from build123d import *

# Parameters (mm, degrees)
SKETCH1_W           = 110
SKETCH1_H           = 30
BOSS_EXTRUDE1_DEPTH = 6
SKETCH2_R           = 2
CUT_EXTRUDE1_DEPTH  = 10


with BuildPart() as part:
    # Sketch1 → Boss-Extrude1 (new body)
    with BuildSketch(Plane(origin=(0, 0, 0), x_dir=(1, 0, 0), z_dir=(0, 1, 0))):
        with Locations((-47.510460251, 50.167364017)):
            Rectangle(SKETCH1_W, SKETCH1_H)
    extrude(amount=BOSS_EXTRUDE1_DEPTH)

    # Sketch2 → Cut-Extrude1 (cut)
    with BuildSketch(Plane.XZ):
        with Locations((-72.510460251, -61.167364017)):
            Circle(SKETCH2_R)
        with Locations((-47.510460251, -61.167364017)):
            Circle(SKETCH2_R)
        with Locations((-22.510460251, -61.167364017)):
            Circle(SKETCH2_R)
        with Locations((-17.510460251, -43.167364017)):
            Circle(SKETCH2_R)
        with Locations((-37.510460251, -43.167364017)):
            Circle(SKETCH2_R)
    extrude(amount=-CUT_EXTRUDE1_DEPTH, mode=Mode.SUBTRACT)


solid = part.part
Input: part model. Units: mm. Frame: model coordinates. Give positions to 0.01 mm unless a question says otherwise; leave off trailing zeros. Loops run counter-clockwise (first coordinate to the right, second up) from the corner with the lowest first, then second, coordinate; pieces in that order, holes last. Notation, with made-up numbers: (63.25, 15.5) -> (80.25, 15.5) arc R6 ccw to (80.25, 20.5) -> close; hole circle Ø1 at (32.25, 30). An arc over 180 degrees is marked (long way). Answer as a JSON object with one key per item and string values. Group by question number.
Item 1: Cut plane C-C, the plane y = 4.15. Return the cut outline in (x, z).
Item 2: Line query: probe 1 along X at (y, z) = (0.9, -59.5); probe 2 along X at (y, z) = (4.2, -42.5); probe 3 along Z at (x, y) = (-72.5, 5.6). Output: solid intervals per line, ascending.
Item 3: Pull-direction query (X, two-part tool) for faces 1 (the flat face through (-102.51, 3, -50)), 2 (the cylindrical face through (-49.51, 2.96, -61.08)), 3 (the flat face through (-48, 6, -50)); classes: released by +X, released by -X, zero draft, split by the parting line, or undercut.
Item 4: Cut plane A-A, the plane z = -44.25. Return the cut outline in (x, y), and give its area (3 significant figures).
Item 5: Cut plane B-B, the plane x = -37. Return the cut outline in (y, z), and give its area (3 significant figures).
Checks:
{
 "1": {"outline": "(-102.51, -65.17) -> (7.49, -65.17) -> (7.49, -35.17) -> (-102.51, -35.17) -> close; hole circle Ø4 at (-72.51, -61.17); hole circle Ø4 at (-47.51, -61.17); hole circle Ø4 at (-37.51, -43.17); hole circle Ø4 at (-22.51, -61.17); hole circle Ø4 at (-17.51, -43.17)"},
 "2": {"probe 1": "x = -102.51 to -73.61, -71.41 to -48.61, -46.41 to -23.61, -21.41 to 7.49", "probe 2": "x = -102.51 to -39.4, -35.63 to -19.4, -15.63 to 7.49", "probe 3": "z = -65.17 to -63.17, -59.17 to -35.17"},
 "3": {"face 1": "released by -X", "face 2": "undercut", "face 3": "zero draft"},
 "4": {"outline": "(-102.51, 0) -> (-39.19, 0) -> (-39.19, 6) -> (-102.51, 6) -> close; (-35.83, 0) -> (-19.19, 0) -> (-19.19, 6) -> (-35.83, 6) -> close; (-15.83, 0) -> (7.49, 0) -> (7.49, 6) -> (-15.83, 6) -> close", "area": "620 mm²"},
 "5": {"outline": "(0, -65.17) -> (6, -65.17) -> (6, -45.1) -> (0, -45.1) -> close; (0, -41.23) -> (6, -41.23) -> (6, -35.17) -> (0, -35.17) -> close", "area": "157 mm²"}
}
